Verification items for the finished model (mm, model axes). Coordinates: 2 decimals unless noted, no trailing zeros. Order: outer loops, then holes, each group sorted by start corner. A loop starts at its lowest first (then second) coordinate and runs counter-clockwise, first axis right, second up. Notation, with made-up numbers: M -2,74.5 L 11,74.5 A33 ccw 11,105.5 Z; hole C 67.25,30 d4. An arc over 180 degrees is marked long. Write item = value, one per line.
```python
from build123d import *

# Parameters (mm, degrees)
SKETCH_1_W          = 60
SKETCH_1_H          = 50
EXTRUDE_1_DEPTH     = 3
SKETCH_7_R          = 1.05
CUT_EXTRUDE_1_DEPTH = 10
SKETCH_8_R          = 1.55
CUT_EXTRUDE_2_DEPTH = 10
FILLET_1_R          = 12


with BuildPart() as part:
    # 草图1 → 凸台-拉伸1 (new body)
    with BuildSketch(Plane(origin=(0, 0, 0), x_dir=(1, 0, 0), z_dir=(0, 1, 0))):
        Rectangle(SKETCH_1_W, SKETCH_1_H)
    extrude(amount=EXTRUDE_1_DEPTH)

    # 草图7 → 切除-拉伸1 (cut)
    with BuildSketch(Plane(origin=(0, 3, 0), x_dir=(1, 0, 0), z_dir=(0, 1, 0))):
        with Locations((13.5, 10)):
            Circle(SKETCH_7_R)
        with Locations((-13.5, 10)):
            Circle(SKETCH_7_R)
        with Locations((-13.5, -10)):
            Circle(SKETCH_7_R)
        with Locations((13.5, -10)):
            Circle(SKETCH_7_R)
    extrude(amount=-CUT_EXTRUDE_1_DEPTH, mode=Mode.SUBTRACT)

    # 草图8 → 切除-拉伸2 (cut)
    with BuildSketch(Plane.XZ):
        with Locations((27, 8)):
            Circle(SKETCH_8_R)
        with Locations((10, 22)):
            Circle(SKETCH_8_R)
        with Locations((-10, 22)):
            Circle(SKETCH_8_R)
        with Locations((-27, 8)):
            Circle(SKETCH_8_R)
        with Locations((-27, -8)):
            Circle(SKETCH_8_R)
        with Locations((-10, -22)):
            Circle(SKETCH_8_R)
        with Locations((10, -22)):
            Circle(SKETCH_8_R)
        with Locations((27, -8)):
            Circle(SKETCH_8_R)
    extrude(amount=-CUT_EXTRUDE_2_DEPTH, mode=Mode.SUBTRACT)

    # 圆角1
    fillet_1_edges = [part.edges().sort_by_distance(p)[0] for p in [
        (30, 1.5, 25),
        (-30, 1.5, 25),
        (-30, 1.5, -25),
        (30, 1.5, -25),
    ]]
    fillet(fillet_1_edges, radius=FILLET_1_R)


solid = part.part
```
Item 1: Sectioned sample at C-C, the plane y = 1.25. Give the number of separate pieces and of enclosed holes in the cut face, then the cut area to 3 significant figures.
Report:
separate_pieces = 1
enclosed_holes = 12
area = 2,800 mm^2
Item 2: Gauge pin test, flat end, axial feed: pin 1 (1 mm diameter, centred on y = 0.5, z = -15.5, fed in from +X). Record the tip position at first contact, or that the pin passes through.
Report:
pin_1 = 29.83
Item 3: Scan lines: L1, parallel to Z at x = -10, y = 1.85; L2, parallel to Z at x = 13.5, y = 1.15; L3, parallel to X at y = 1.35, z = 10. Record each from-to range of solid material in increasing order. Write a range as from..to.
Report:
L1 = -25..-23.55, -20.45..20.45, 23.55..25
L2 = -25..-11.05, -8.95..8.95, 11.05..25
L3 = -30..-14.55, -12.45..12.45, 14.55..30
Item 4: Release check for a two-part mould opening along X. For faces 1 (the flat face through (0, 1, 25)), 2 (the cylindrical face through (26.39, 1.52, 21.58)), 3 (the cylindrical face through (28.432, 1.479, 7.406)) record: pulls with the +X half, pulls with the -X half, needs draft (parallel to the pull), parting line crosses it, or undercut.
Report:
face_1 = needs draft
face_2 = pulls with the +X half
face_3 = undercut
Item 5: Sectioned sample at A-A, the plane z = 8. Enter the section's corners in (x, y), then the cut area to 3 significant figures.
Report:
outline = M -30,0 L -28.55,0 L -28.55,3 L -30,3 Z; M -25.45,0 L 25.45,0 L 25.45,3 L -25.45,3 Z; M 28.55,0 L 30,0 L 30,3 L 28.55,3 Z
area = 161 mm^2
Item 6: Sectioned sample at B-B, the plane x = 10. Enter the section's corners in (y, z).
Report:
outline = M 0,-25 L 3,-25 L 3,-23.55 L 0,-23.55 Z; M 0,-20.45 L 3,-20.45 L 3,20.45 L 0,20.45 Z; M 0,23.55 L 3,23.55 L 3,25 L 0,25 Z
